Input: part model. Units: mm. Frame: model coordinates. Give positions to 0.01 mm unless a question says otherwise; leave off trailing zeros. Write each loop counter-clockwise with the first axis right and the second up, starting at its lowest first coordinate (ties: lowest second). Pieces come first, ordered by that corner, then holes.
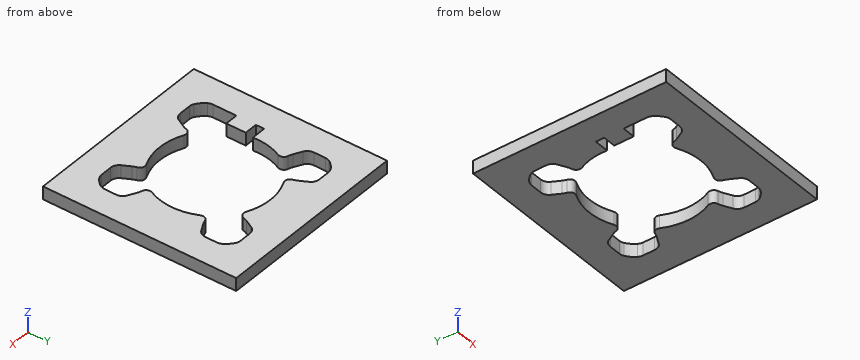
Autodesk Inventor part; units mm, degrees
ref_plane "YZ Plane" through (0, 0, 0) normal (1, 0, 0) x (0, 1, 0)
ref_plane "XZ Plane" through (0, 0, 0) normal (0, 1, 0) x (-1, 0, 0)
ref_plane "XY Plane" through (0, 0, 0) normal (0, 0, 1) x (1, 0, 0)
ref_plane "Work Plane1" through (0, 0, 0) normal (0, 0, 1) x (1, 0, 0)
sketch "Sketch1" plane through (0, 0, 0) normal (0, 0, 1) x (1, 0, 0)
  circle A0 centre (0, 0) radius 8
  arc A1 (-21.8566, 27) -> (-23.5705, 26.52) centre (-21.8566, 23.7) ccw
  line L0 (-21.8566, 27) -> (-17.3137, 27)
  arc A2 (-14.4021, 25.2532) -> (-17.3137, 27) centre (-17.3137, 23.7) ccw
  line L1 (-14.4021, 25.2532) -> (-12.8239, 22.2947)
  arc A3 (-12.2013, 20.6664) -> (-12.8239, 22.2947) centre (-19, 19) ccw
  arc A4 (-12.2013, 20.6664) -> (-9.3857, 19.3432) centre (-10.2588, 21.1426) ccw
  arc A5 (9.3857, 19.3432) -> (-9.3857, 19.3432) centre (0, 0) ccw
  arc A6 (9.3857, 19.3432) -> (12.2013, 20.6664) centre (10.2588, 21.1426) ccw
  arc A7 (12.8239, 22.2947) -> (12.2013, 20.6664) centre (19, 19) ccw
  line L2 (12.8239, 22.2947) -> (14.4021, 25.2532)
  arc A8 (17.3137, 27) -> (14.4021, 25.2532) centre (17.3137, 23.7) ccw
  line L3 (17.3137, 27) -> (21.8566, 27)
  arc A9 (23.5705, 26.52) -> (21.8566, 27) centre (21.8566, 23.7) ccw
  arc A10 (26.52, 23.5705) -> (23.5705, 26.52) centre (19, 19) ccw
  arc A11 (27, 21.8566) -> (26.52, 23.5705) centre (23.7, 21.8566) ccw
  line L4 (27, 21.8566) -> (27, 17.3137)
  arc A12 (25.2532, 14.4021) -> (27, 17.3137) centre (23.7, 17.3137) ccw
  line L5 (25.2532, 14.4021) -> (22.2947, 12.8239)
  arc A13 (20.6664, 12.2013) -> (22.2947, 12.8239) centre (19, 19) ccw
  arc A14 (20.6664, 12.2013) -> (19.3432, 9.3857) centre (21.1426, 10.2588) ccw
  arc A15 (19.3432, -9.3857) -> (19.3432, 9.3857) centre (0, 0) ccw
  arc A16 (19.3432, -9.3857) -> (20.6664, -12.2013) centre (21.1426, -10.2588) ccw
  arc A17 (22.2947, -12.8239) -> (20.6664, -12.2013) centre (19, -19) ccw
  line L6 (22.2947, -12.8239) -> (25.2532, -14.4021)
  arc A18 (27, -17.3137) -> (25.2532, -14.4021) centre (23.7, -17.3137) ccw
  line L7 (27, -17.3137) -> (27, -21.8566)
  arc A19 (26.52, -23.5705) -> (27, -21.8566) centre (23.7, -21.8566) ccw
  arc A20 (23.5705, -26.52) -> (26.52, -23.5705) centre (19, -19) ccw
  arc A21 (21.8566, -27) -> (23.5705, -26.52) centre (21.8566, -23.7) ccw
  line L8 (21.8566, -27) -> (17.3137, -27)
  arc A22 (14.4021, -25.2532) -> (17.3137, -27) centre (17.3137, -23.7) ccw
  line L9 (14.4021, -25.2532) -> (12.8239, -22.2947)
  arc A23 (12.2013, -20.6664) -> (12.8239, -22.2947) centre (19, -19) ccw
  arc A24 (12.2013, -20.6664) -> (9.3857, -19.3432) centre (10.2588, -21.1426) ccw
  arc A25 (-9.3857, -19.3432) -> (9.3857, -19.3432) centre (0, 0) ccw
  arc A26 (-9.3857, -19.3432) -> (-12.2013, -20.6664) centre (-10.2588, -21.1426) ccw
  arc A27 (-12.8239, -22.2947) -> (-12.2013, -20.6664) centre (-19, -19) ccw
  line L10 (-12.8239, -22.2947) -> (-14.4021, -25.2532)
  arc A28 (-17.3137, -27) -> (-14.4021, -25.2532) centre (-17.3137, -23.7) ccw
  line L11 (-17.3137, -27) -> (-21.8566, -27)
  arc A29 (-23.5705, -26.52) -> (-21.8566, -27) centre (-21.8566, -23.7) ccw
  arc A30 (-26.52, -23.5705) -> (-23.5705, -26.52) centre (-19, -19) ccw
  arc A31 (-27, -21.8566) -> (-26.52, -23.5705) centre (-23.7, -21.8566) ccw
  line L12 (-27, -21.8566) -> (-27, -12.7696)
  line L13 (-27, -12.7696) -> (-22, -12.7696)
  line L14 (-22, -12.7696) -> (-22, -5.2304)
  line L15 (-22, -5.2304) -> (-27, -5.2304)
  line L16 (-27, -5.2304) -> (-27, -2)
  line L17 (-27, -2) -> (-21.4068, -2)
  arc A32 (-19.3432, 9.3857) -> (-21.4068, -2) centre (0, 0) ccw
  arc A33 (-19.3432, 9.3857) -> (-20.6664, 12.2013) centre (-21.1426, 10.2588) ccw
  arc A34 (-22.2947, 12.8239) -> (-20.6664, 12.2013) centre (-19, 19) ccw
  line L18 (-22.2947, 12.8239) -> (-25.2532, 14.4021)
  arc A35 (-27, 17.3137) -> (-25.2532, 14.4021) centre (-23.7, 17.3137) ccw
  line L19 (-27, 17.3137) -> (-27, 21.8566)
  arc A36 (-26.52, 23.5705) -> (-27, 21.8566) centre (-23.7, 21.8566) ccw
  arc A37 (-23.5705, 26.52) -> (-26.52, 23.5705) centre (-19, 19) ccw
  line L20 (42.5, 37.5) -> (42.5, -37.5)
  line L21 (42.5, -37.5) -> (37.5, -37.5)
  line L22 (37.5, -37.5) -> (37.5, 37.5)
  line L23 (37.5, 37.5) -> (42.5, 37.5)
  line L24 (-42.5, -37.5) -> (-42.5, 37.5)
  line L25 (-42.5, 37.5) -> (-37.5, 37.5)
  line L26 (-37.5, 37.5) -> (-37.5, -37.5)
  line L27 (-37.5, -37.5) -> (-42.5, -37.5)
  line L28 (-37.5, -37.5) -> (37.5, -37.5)
  line L29 (-37.5, 37.5) -> (37.5, 37.5)
  point P0 (0, 0)
extrude "Extrusion1" add sketch "Sketch1" along normal blind 5 contours L22 L28 L26 L29
properties part number "Soporte Cilindro Cortadora"
Item 1: Section B-B (x = 7). Return loops of the section in (y, z).
Item 2: Section A-A (y = -11). Return loops of the section in (x, z).
Item 3: Ray query, line 1 (X direction, y = -19, z = 1.2); line 2 (Y direction, x = 17, z = 1.75); line 3 (Y direction, x = 22, z = 2.05). Return the intervals inside material, ascending.
Solved:
1. outline: (-37.5, 0) - (-20.33, 0) - (-20.33, 5) - (-37.5, 5) - close; (20.33, 0) - (37.5, 0) - (37.5, 5) - (20.33, 5) - close
2. outline: (-37.5, 0) - (-22, 0) - (-22, 5) - (-37.5, 5) - close; (19.28, 0) - (37.5, 0) - (37.5, 5) - (19.28, 5) - close
3. line 1: x = -37.5 to -27, 27 to 37.5
3. line 2: y = -37.5 to -26.99, 26.99 to 37.5
3. line 3: y = -37.5 to -27, -12.68 to 12.68, 27 to 37.5
